Design review of the part built by this model. Coordinates are the model's own, in mm. Face numbers are marked on the shaded views. Give positions to 0.01 mm unless a question says otherwise; leave off trailing zeros. Loops run counter-clockwise (first coordinate to the right, second up) from the corner with the lowest first, then second, coordinate; pieces in that order, holes last. Notation, with made-up numbers: (-8.75, -23.5) -> (50.25, -23.5) arc R20 cw to (50.25, -9.5) -> close; hole circle Ø3 at (-27, -29). An arc over 180 degrees is marked (long way). Use a Markdown table: item, result. Add a question column.
1. Add section D-D (x = -6.25). State the section outline as (y, z) points, and give its area (3 significant figures).
2. To check wall thickness, follow line 1 (Y direction, x = -4, z = -21.5); line 2 (Z direction, x = -3.5, y = 36); line 3 (Z direction, x = -11.25, y = 36). State the ranges of each line that lie inside material, in increasing order.
3. For pin 1 Ø12 at (y, z) = (-35, -19.5) entering from -X; pin 2 Ø7 at (y, z) = (36, -21.5) entering from -X, all flat-tipped, find the tip position at first contact; note any pin that passes through.
4. Add section A-A (z = -39.5). State the section outline as (x, y) points, and give its area (3 significant figures).
5. Add section B-B (x = -1.5). State the section outline as (y, z) points.
6. Draft analysis for pull direction Z (two halves, no side actions). For the marked faces 1, 2, 3 and 4, state which applies: pulls with the +Z half, pulls with the -Z half, needs draft (parallel to the pull), parting line crosses it, or undercut.
7. Add section C-C (y = -36). State the section outline as (x, z) points.
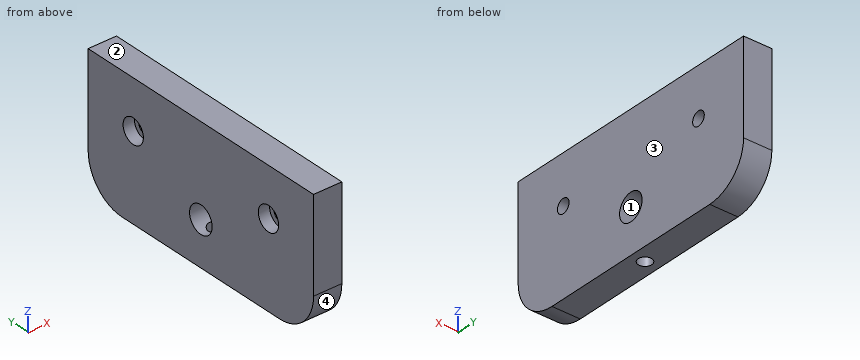
```python
from build123d import *

# Parameters (mm, degrees)
SKETCH_R        = 6
SKETCH_R_2      = 3.1
PAD_DEPTH       = 12.5
SKETCH001_R     = 5.4
POCKET_DEPTH    = 5
SKETCH003_R     = 3
POCKET001_DEPTH = 15


with BuildPart() as part:
    # Sketch → Pad (new body)
    with BuildSketch(Plane(origin=(0, 0, 0), x_dir=(0, -1, 0), z_dir=(-1, 0, 0))):
        with BuildLine():
            Line((-60, 0), (60, 0))
            Line((60, 0), (60, -41))
            ThreePointArc((42, -59), (54.727922, -53.727922), (60, -41))
            Line((42, -59), (-42.000001, -59))
            ThreePointArc((-60, -41.000038), (-54.727909, -53.727935), (-42.000001, -59))
            Line((-60, -41.000038), (-60, 0))
        make_face()
        with Locations((0, -39.5)):
            Circle(SKETCH_R, mode=Mode.SUBTRACT)
        with Locations((-36, -21.5)):
            Circle(SKETCH_R_2, mode=Mode.SUBTRACT)
        with Locations((36, -21.5)):
            Circle(SKETCH_R_2, mode=Mode.SUBTRACT)
    extrude(amount=PAD_DEPTH)

    # Sketch001 → Pocket (cut)
    with BuildSketch(Plane(origin=(-12.5, 0, 0), x_dir=(0, -1, 0), z_dir=(-1, 0, 0))):
        with Locations((-36, -21.5)):
            Circle(SKETCH001_R)
        with Locations((36, -21.5)):
            Circle(SKETCH001_R)
    extrude(amount=-POCKET_DEPTH, mode=Mode.SUBTRACT)

    # Sketch003 → Pocket001 (cut)
    with BuildSketch(Plane(origin=(0, 0, -59), x_dir=(0, -1, 0), z_dir=(0, 0, -1))):
        with Locations((0, 6.25)):
            Circle(SKETCH003_R)
    extrude(amount=-POCKET001_DEPTH, mode=Mode.SUBTRACT)


solid = part.part
```
Taken from the geometry:
| question | item | result |
|---|---|---|
| 1 | outline | (-60, -41) arc R18 ccw to (-42, -59) -> (-3, -59) -> (-3, -44.7) arc R6 cw (long way) to (3, -44.7) -> (3, -59) -> (42, -59) arc R18 ccw to (60, -41) -> (60, 0) -> (-60, 0) -> close; hole circle Ø6.2 at (-36, -21.5); hole circle Ø6.2 at (36, -21.5) |
| 1 | area | 6,680 mm^2 |
| 2 | line 1 | y = -60 to -39.1, -32.9 to 32.9, 39.1 to 60 |
| 2 | line 2 | z = -59 to -24.6, -18.4 to 0 |
| 2 | line 3 | z = -59 to -26.9, -16.1 to 0 |
| 3 | pin 1 | stops at x = -12.5 |
| 3 | pin 2 | stops at x = -7.5 |
| 4 | outline | (-12.5, -60) -> (0, -60) -> (0, -6) -> (-12.5, -6) -> close; (-12.5, 6) -> (0, 6) -> (0, 60) -> (-12.5, 60) -> close |
| 4 | area | 1,350 mm^2 |
| 5 | outline | (-60, -41) arc R18 ccw to (-42, -59) -> (42, -59) arc R18 ccw to (60, -41) -> (60, 0) -> (-60, 0) -> close; hole circle Ø6.2 at (-36, -21.5); hole circle Ø12 at (0, -39.5); hole circle Ø6.2 at (36, -21.5) |
| 6 | face 1 | undercut |
| 6 | face 2 | pulls with the +Z half |
| 6 | face 3 | needs draft |
| 6 | face 4 | pulls with the -Z half |
| 7 | outline | (-12.5, -59) -> (0, -59) -> (0, -24.6) -> (-7.5, -24.6) -> (-7.5, -26.9) -> (-12.5, -26.9) -> close; (-12.5, -16.1) -> (-7.5, -16.1) -> (-7.5, -18.4) -> (0, -18.4) -> (0, 0) -> (-12.5, 0) -> close |
